Check sheet for the modelled part. Datum: model origin and axes. Units: mm. A direction names the side the tool comes from. Round coordinates to 2 decimals unless told otherwise and drop trailing zeros. Loops run counter-clockwise (first coordinate to the right, second up) from the corner with the lowest first, then second, coordinate; pieces in that order, holes last. Notation, with made-up numbers: (86, -35.5) - (103, -35.5) arc R30 cw to (103, -10.5) - close; hole circle Ø10 at (12.25, 76). An arc over 180 degrees is marked (long way). Put each result on its own line as item: value. Start each with the question number.
Item 1: Tool access check on faces 1 (the flat face through (0, 1.71, -4)), 2 (the flat face through (-5.35, -1, -10)), 3 (the flat face through (0, 10, 0)). Record the directions out of +Z, -Z, +X, -X, +Y, -Y that give a thin tool (end or side, any length) a straight path to the whole face; none if there is none.
Item 2: Gauge pin test, flat ends, axial feed: pin 1 Ø4 at (x, z) = (-1, -4) entering from -Y; pin 2 Ø0.6 at (x, y) = (-5.5, -2) entering from -Z; pin 3 Ø6 at (x, z) = (-3.5, -14) entering from -Y. Record the tip position at first contact, or that the pin passes through.
Item 3: Section check C-C, the plane z = -9.25. Record the cut outline in (x, y).
Item 4: Draft check along X on faces 4 (the flat face through (0, 6.363, -4)), 5 (the flat face through (0, 10.9, -8)), 6 (the flat face through (-6.05, 5, -8)), 7 (the flat face through (-3.718, 8.997, -3.944)). Enter one of: pulls with the +X half, pulls with the -X half, needs draft (parallel to the pull), parting line crosses it, or undercut.
Item 5: Section check B-B, the plane x = 0.5. Record the cut outline in (y, z).
Item 6: Section check A-A, the plane z = -7. Give the number of separate pieces and of enclosed holes in the cut face, and give its area (4 significant figures).
Item 7: Section check D-D, the plane x = -1.25. Record the cut outline in (y, z).
Item 8: Material ranges on line 1 along Y through (x, z) = (-1, -6.25); line 2 along Y through (x, z) = (-1.5, -1); line 3 along X through (y, z) = (3.5, -6.5) (3 decimals), recorded low to high.
Autodesk Inventor part; units mm, degrees
ref_plane "YZ Plane" through (0, 0, 0) normal (1, 0, 0) x (0, 1, 0)
ref_plane "XZ Plane" through (0, 0, 0) normal (0, 1, 0) x (-1, 0, 0)
ref_plane "XY Plane" through (0, 0, 0) normal (0, 0, 1) x (1, 0, 0)
sketch "Sketch1" plane through (0, 0, 0) normal (0, 0, 1) x (1, 0, 0)
  line L0 (-6.05, 10.9) -> (6.05, 10.9)
  line L1 (6.05, 10.9) -> (6.05, 0.3)
  line L2 (6.05, 0.3) -> (-6.05, 0.3)
  line L3 (-6.05, 0.3) -> (-6.05, 10.9)
  point P0 (0, 0)
  dimension "d0" = 10.6
  dimension "d1" = 0.3
  dimension "d2" = 12.1
  dimension "d3" = 6.05
extrude "Extrusion1" add sketch "Sketch1" against normal blind 16.5
sketch "Sketch2" plane through (-6.05, 0.3, 0) normal (0, -1, 0) x (1, 0, 0)
  line L0 (9.4241, -4.8692) -> (1.7869, -4.8692)
  line L1 (1.7869, -4.8692) -> (1.7869, -15.7795)
  line L2 (1.7869, -15.7795) -> (9.4241, -15.7795)
  line L3 (9.4241, -15.7795) -> (9.4241, -4.8692)
  point P0 (6.05, 0)
extrude "Extrusion2" add sketch "Sketch2" along normal blind 0.3
sketch "Sketch3" plane through (-6.05, 0, 0) normal (0, -1, 0) x (1, 0, 0)
  circle A0 centre (4.8, -15.01) radius 0.3
  circle A1 centre (7.3, -15.01) radius 0.3
  circle A2 centre (4.8, -13.01) radius 0.3
  circle A3 centre (7.3, -13.01) radius 0.3
  line L0 (12.1, 0) -> (0, 0)
  point P0 (6.05, 0)
  dimension "d8" = 1.25
  dimension "d9" = 1.25
  dimension "d10" = 0
  dimension "d11" = 0
  dimension "d12" = 2
  dimension "d13" = 0
  dimension "d14" = 0
  dimension "d15" = 13.01
  dimension "d16" = 0.6
  dimension "d17" = 0.6
  dimension "d18" = 0.6
  dimension "d19" = 0.6
extrude "Extrusion3" add sketch "Sketch3" along normal blind 2.8
sketch "Sketch4" plane through (-6.05, 0.3, 0) normal (0, -1, 0) x (1, 0, 0)
  line L0 (12.1, 0) -> (12.1, -16.5)
  line L1 (12.1, -9) -> (11.4, -9)
  line L2 (11.4, -9) -> (11.4, -11.6)
  line L3 (11.4, -11.6) -> (12.1, -11.6)
  line L4 (12.1, -11.6) -> (12.1, -9)
  line L5 (0, 0) -> (0, -16.5)
  line L6 (0, -9) -> (0.7, -9)
  line L7 (0.7, -9) -> (0.7, -11.6)
  line L8 (0.7, -11.6) -> (0, -11.6)
  line L9 (0, -11.6) -> (0, -9)
  line L10 (12.1, 0) -> (0, 0)
  point P0 (6.05, 0)
  dimension "d22" = 2.6
  dimension "d23" = 2.6
  dimension "d24" = 9
  dimension "d25" = 0
  dimension "d26" = 0.7
  dimension "d27" = 0.7
extrude "Extrusion4" add sketch "Sketch4" along normal blind 3.6
sketch "Sketch5" plane through (0, 0, 0) normal (0, 0, 1) x (1, 0, 0)
  line L0 (-4.225, 1.71) -> (4.225, 1.71)
  line L1 (4.225, 1.71) -> (4.225, 9.49)
  line L2 (4.225, 9.49) -> (-4.225, 9.49)
  line L3 (-4.225, 9.49) -> (-4.225, 1.71)
  line L4 (6.05, 0.3) -> (-6.05, 0.3)
  line L5 (-3.225, 9.49) -> (-4.225, 8.49)
  line L6 (3.225, 9.49) -> (4.225, 8.49)
  point P0 (0, 0)
  dimension "d30" = 7.78
  dimension "d31" = 8.45
  dimension "d32" = 4.225
  dimension "d33" = 1.41
  dimension "d34" = 45
  dimension "d35" = 45
  dimension "d36" = 1
  dimension "d37" = 1
extrude "Extrusion5" cut sketch "Sketch5" against normal blind 8 contours L3 L5 L2 L6 L1 L0
sketch "Sketch6" plane through (0, 0, -8) normal (0, 0, 1) x (1, 0, 0)
  line L0 (-2.6112, 6.3628) -> (2.6965, 6.3628)
  line L1 (2.6965, 6.3628) -> (2.6965, 4.1886)
  line L2 (2.6965, 4.1886) -> (-2.6112, 4.1886)
  line L3 (-2.6112, 4.1886) -> (-2.6112, 6.3628)
  point P0 (0, 0)
extrude "Extrusion6" add sketch "Sketch6" along normal blind 8
properties part number "USB-B"
Check result:
1. face 1: +Z
1. face 2: +Z, -Z, -Y
1. face 3: +Z, +X, -X, +Y, -Y
2. pin 1: y = 0
2. pin 2: z = -11.6
2. pin 3: y = -2.8
3. outline: (-6.05, -3.3) - (-5.35, -3.3) - (-5.35, 0.3) - (-4.26, 0.3) - (-4.26, 0) - (3.37, 0) - (3.37, 0.3) - (5.35, 0.3) - (5.35, -3.3) - (6.05, -3.3) - (6.05, 10.9) - (-6.05, 10.9) - close
4. face 4: undercut
4. face 5: needs draft
4. face 6: pulls with the -X half
4. face 7: undercut
5. outline: (0, -15.78) - (0.3, -15.78) - (0.3, -16.5) - (10.9, -16.5) - (10.9, 0) - (9.49, 0) - (9.49, -8) - (6.36, -8) - (6.36, 0) - (4.19, 0) - (4.19, -8) - (1.71, -8) - (1.71, 0) - (0.3, 0) - (0.3, -4.87) - (0, -4.87) - close
6. separate pieces: 2
6. enclosed holes: 1
6. area: 77.35 mm²
7. outline: (-2.8, -15.31) - (0, -15.31) - (0, -15.78) - (0.3, -15.78) - (0.3, -16.5) - (10.9, -16.5) - (10.9, 0) - (9.49, 0) - (9.49, -8) - (6.36, -8) - (6.36, 0) - (4.19, 0) - (4.19, -8) - (1.71, -8) - (1.71, 0) - (0.3, 0) - (0.3, -4.87) - (0, -4.87) - (0, -12.71) - (-2.8, -12.71) - (-2.8, -13.31) - (0, -13.31) - (0, -14.71) - (-2.8, -14.71) - close
8. line 1: 0 to 1.71, 4.19 to 6.36, 9.49 to 10.9
8. line 2: 0.3 to 1.71, 4.19 to 6.36, 9.49 to 10.9
8. line 3: -6.05 to -4.225, 4.225 to 6.05
